from build123d import *

# Parameters (mm, degrees)
SKETCH_1_R          = 11
EXTRUDE_1_DEPTH     = 2
SKETCH_2_R          = 9.17
EXTRUDE_2_DEPTH     = 11
SKETCH_3_R          = 11
EXTRUDE_3_DEPTH     = 2
SKETCH_4_R          = 2.5
CUT_EXTRUDE_1_DEPTH = 26
SKETCH_5_R          = 7.5
SKETCH_5_R_2        = 2.5
EXTRUDE_4_DEPTH     = 8


with BuildPart() as part:
    # 草图1 → 凸台-拉伸1 (new body)
    with BuildSketch(Plane(origin=(0, 0, 0), x_dir=(1, 0, 0), z_dir=(0, 1, 0))):
        with Locations(Location((0, 0, 0), (0, 0, 270))):
            Circle(SKETCH_1_R)
    extrude(amount=EXTRUDE_1_DEPTH)

    # 草图2 → 凸台-拉伸2 (add)
    with BuildSketch(Plane(origin=(0, 2, 0), x_dir=(1, 0, 0), z_dir=(0, 1, 0))):
        with Locations(Location((0, 0, 0), (0, 0, 270))):
            Circle(SKETCH_2_R)
    extrude(amount=EXTRUDE_2_DEPTH)

    # 草图3 → 凸台-拉伸3 (add)
    with BuildSketch(Plane(origin=(0, 13, 0), x_dir=(1, 0, 0), z_dir=(0, 1, 0))):
        with Locations(Location((0, 0, 0), (0, 0, 270))):
            Circle(SKETCH_3_R)
    extrude(amount=EXTRUDE_3_DEPTH)

    # 草图4 → 切除-拉伸1 (cut)
    with BuildSketch(Plane(origin=(0, 15, 0), x_dir=(1, 0, 0), z_dir=(0, 1, 0))):
        with Locations(Location((0, 0, 0), (0, 0, 270))):
            Circle(SKETCH_4_R)
    extrude(amount=-CUT_EXTRUDE_1_DEPTH, mode=Mode.SUBTRACT)

    # 草图5 → 凸台-拉伸4 (add)
    with BuildSketch(Plane.XZ):
        with Locations(Location((0, 0, 0), (0, 0, 270))):
            Circle(SKETCH_5_R)
        with Locations(Location((0, 0, 0), (0, 0, 90))):
            Circle(SKETCH_5_R_2, mode=Mode.SUBTRACT)
    extrude(amount=EXTRUDE_4_DEPTH)


solid = part.part
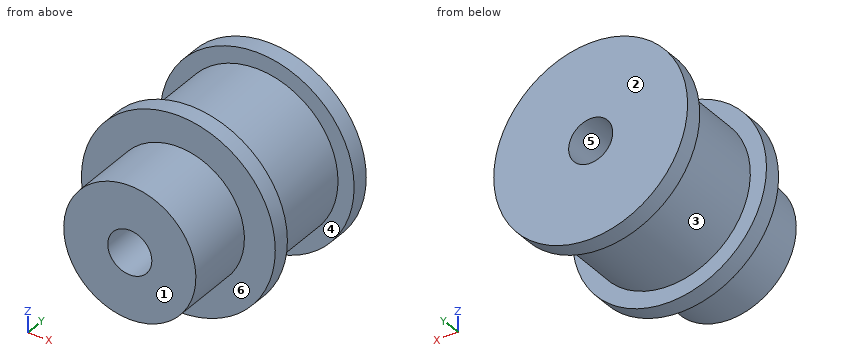
CAD build for the part. Positions are in the model's coordinates, mm. Face numbers are marked on the shaded views. A direction names the side the tool comes from. Coordinates: 2 decimals unless noted, no trailing zeros. Write each loop counter-clockwise with the first axis right and the second up, starting at its lowest first coordinate (ties: lowest second). Pieces come first, ordered by that corner, then holes. Notation, with made-up numbers: M 77.25,-7.75 L 107.25,-7.75 A20 ccw 107.25,25.25 Z; hole C 81,6 d8. An arc over 180 degrees is marked long. Answer as a JSON object with one key per item and string values. Group by question number.
1) Saw through at A-A (z = 0). Write the cut outline in (x, y), plus the area to 3 significant figures.
2) Wall check: line 1 (X direction, y = 3, z = 0); line 2 (X direction, y = -0.75, z = 0); line 3 (Y direction, x = 6.25, z = -5). Give the ranges that are in metal, low to high. Write a range as from..to.
3) Pin check, flat tips, straight feed: pin 1 Ø5 at (y, z) = (11, -3.5) entering from +X; pin 2 Ø1.5 at (y, z) = (-1, 3.5) entering from +X; pin 3 Ø5 at (x, y) = (-4, -2) entering from -Z. Stop position of each tip, or through.
4) Mould opens along Y. For the marked faces 1, 2 and 3 say: +Y half, -Y half, draft (parallel to the pull), parting line (faces both ways), or undercut.
5) Saw through at C-C (y = -6.25). Write the cut outline in (x, z), plus the area to 3 significant figures.
6) Saw through at B-B (x = 0). Write the cut outline in (y, z).
7) Saw through at D-D (x = 8.75). Write the cut outline in (y, z), plus the area to 3 significant figures.
8) Tool access for the marked faces 4, 5 and 6: list every direction of +Z, -Z, +X, -X, +Y, -Y with a clear straight run to the whole face (end or side of a thin tool).
Values follow:
{
 "1": {"outline": "M -11,0 L -7.5,0 L -7.5,-8 L -2.5,-8 L -2.5,15 L -11,15 L -11,13 L -9.17,13 L -9.17,2 L -11,2 Z; M 2.5,-8 L 7.5,-8 L 7.5,0 L 11,0 L 11,2 L 9.17,2 L 9.17,13 L 11,13 L 11,15 L 2.5,15 Z", "area": "295 mm2"},
 "2": {"line 1": "x = -9.17..-2.5, 2.5..9.17", "line 2": "x = -7.5..-2.5, 2.5..7.5", "line 3": "y = 0..15"},
 "3": {"pin 1": "stops at x = 10.82", "pin 2": "stops at x = 6.98", "pin 3": "stops at z = -10.71"},
 "4": {"face 1": "-Y half", "face 2": "+Y half", "face 3": "undercut"},
 "5": {"outline": "C 0,0 d15; hole C 0,0 d5", "area": "157 mm2"},
 "6": {"outline": "M -8,-7.5 L 0,-7.5 L 0,-11 L 2,-11 L 2,-9.17 L 13,-9.17 L 13,-11 L 15,-11 L 15,-2.5 L -8,-2.5 Z; M -8,2.5 L 15,2.5 L 15,11 L 13,11 L 13,9.17 L 2,9.17 L 2,11 L 0,11 L 0,7.5 L -8,7.5 Z"},
 "7": {"outline": "M 0,-6.67 L 2,-6.67 L 2,-2.74 L 13,-2.74 L 13,-6.67 L 15,-6.67 L 15,6.67 L 13,6.67 L 13,2.74 L 2,2.74 L 2,6.67 L 0,6.67 Z", "area": "114 mm2"},
 "8": {"face 4": "none", "face 5": "+Y, -Y", "face 6": "-Y"}
}
